Part model, mm, in its own coordinate system. Face numbers are marked on the shaded views. A direction names the side the tool comes from. Coordinates: 2 decimals unless noted, no trailing zeros. Order: outer loops, then holes, each group sorted by start corner. A loop starts at its lowest first (then second) coordinate and runs counter-clockwise, first axis right, second up.
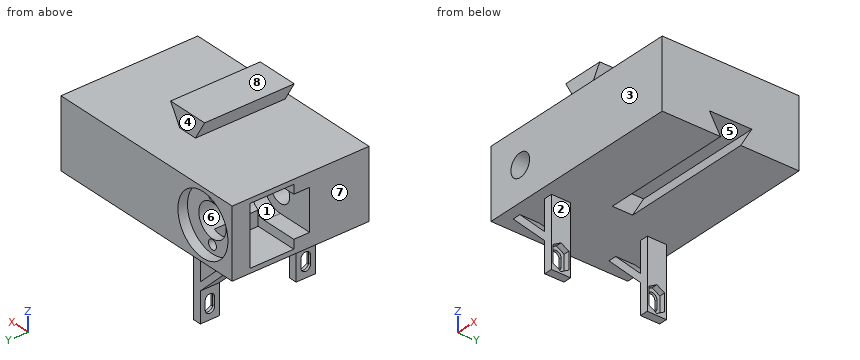
```python
from build123d import *

# Parameters (mm, degrees)
SKETCH1_W                       = 38
SKETCH1_H                       = 50
BOSS_EXTRUDE1_DEPTH             = 25
BOSS_EXTRUDE2_START             = -22.75
BOSS_EXTRUDE2_DEPTH             = 32.75
CUT_EXTRUDE1_DEPTH              = 10
CUT_EXTRUDE2_REACH              = 88.168
CUT_EXTRUDE2_DIRECTION_2_DEPTH  = 87.168439698
SKETCH15_R                      = 11.1
CUT_EXTRUDE8_DEPTH              = 3.5
SKETCH16_R                      = 6.05
CUT_EXTRUDE9_DEPTH              = 19
SKETCH17_R                      = 6.05
CUT_EXTRUDE10_DEPTH             = 5.8
CUT_EXTRUDE11_START             = -16
CUT_EXTRUDE11_DEPTH             = 16
SKETCH19_R                      = 1.75
CUT_EXTRUDE12_DEPTH             = 19
CIRPATTERN1_COUNT               = 2
CIRPATTERN1_ANGLE               = 90
CIRPATTERN1_THE_OTHER_WAY_COUNT = 2
CIRPATTERN1_THE_OTHER_WAY_ANGLE = 90
SKETCH20_R                      = 4.15
CUT_EXTRUDE13_DEPTH             = 58.174207472
SKETCH21_R                      = 1.75
CUT_EXTRUDE14_DEPTH             = 16
SKETCH22_W                      = 3
SKETCH22_H                      = 7
BOSS_EXTRUDE5_DEPTH             = 25
CUT_EXTRUDE15_DEPTH             = 10
CUT_EXTRUDE16_START             = 2.1
CUT_EXTRUDE16_DEPTH             = 2.1
BOSS_EXTRUDE7_DEPTH             = 7
BOSS_EXTRUDE8_DEPTH             = 7


with BuildPart() as part:
    # Sketch1 → Boss-Extrude1 (new body)
    with BuildSketch(Plane.XY):
        with Locations((-19, 0)):
            Rectangle(SKETCH1_W, SKETCH1_H)
    boss_extrude1 = extrude(amount=BOSS_EXTRUDE1_DEPTH)

    # Sketch2 → Boss-Extrude2 (add)
    with BuildSketch(Plane(origin=(0, 0, 0), x_dir=(0, 0, -1), z_dir=(0, 1, 0)).offset(BOSS_EXTRUDE2_START)):
        Polygon((-25, 0), (-25, 3.5), (-32, 7.541451884), (-32, 0), align=None)
    boss_extrude2 = extrude(amount=BOSS_EXTRUDE2_DEPTH)

    # Sketch3 → Cut-Extrude1 (cut)
    with BuildSketch(Plane(origin=(0, 0, 0), x_dir=(0, 0, -1), z_dir=(1, 0, 0))):
        Polygon((0, -3.7), (0, 3.7), (-7, 7.741451884), (-7, -7.741451884), align=None)
    cut_extrude1 = extrude(amount=-CUT_EXTRUDE1_DEPTH, mode=Mode.SUBTRACT)

    # Mirror1: Boss-Extrude1, Boss-Extrude2, Cut-Extrude1 across plane
    add(boss_extrude1.mirror(Plane(origin=(0, 0, 0), x_dir=(0, 0, 1), z_dir=(1, 0, 0))))
    add(boss_extrude2.mirror(Plane(origin=(0, 0, 0), x_dir=(0, 0, 1), z_dir=(1, 0, 0))))
    add(cut_extrude1.mirror(Plane(origin=(0, 0, 0), x_dir=(0, 0, 1), z_dir=(1, 0, 0))), mode=Mode.SUBTRACT)

    # Sketch4 → Cut-Extrude2 (cut, up to next)
    with BuildSketch(Plane(origin=(38, 0, 0), x_dir=(0, 0, -1), z_dir=(1, 0, 0)), mode=Mode.PRIVATE) as cut_extrude2_sk1:
        Polygon((0, -3.7), (0, 3.7), (-7, 7.741451884), (-7, -7.741451884), align=None)
    cut_extrude2_tool1 = extrude(cut_extrude2_sk1.sketch, amount=-CUT_EXTRUDE2_REACH, mode=Mode.PRIVATE) & part.part
    add(cut_extrude2_tool1.solids().sort_by_distance((38, 0, 3.9121))[0], mode=Mode.SUBTRACT)

    # Sketch4 → Cut-Extrude2 direction 2 (cut)
    with BuildSketch(Plane(origin=(38, 0, 0), x_dir=(0, 0, -1), z_dir=(1, 0, 0))):
        Polygon((0, -3.7), (0, 3.7), (-7, 7.741451884), (-7, -7.741451884), align=None)
    extrude(amount=CUT_EXTRUDE2_DIRECTION_2_DEPTH, mode=Mode.SUBTRACT)

    # Sketch15 → Cut-Extrude8 (cut)
    with BuildSketch(Plane(origin=(0, 25, 0), x_dir=(1, 0, 0), z_dir=(0, 1, 0))):
        with Locations(Location((-25, -12.5, 0), (0, 0, 270))):
            Circle(SKETCH15_R)
    extrude(amount=-CUT_EXTRUDE8_DEPTH, mode=Mode.SUBTRACT)

    # Sketch16 → Cut-Extrude9 (cut)
    with BuildSketch(Plane(origin=(0, 21.5, 0), x_dir=(1, 0, 0), z_dir=(0, 1, 0))):
        with Locations(Location((-25, -12.5, 0), (0, 0, 270))):
            Circle(SKETCH16_R)
    extrude(amount=-CUT_EXTRUDE9_DEPTH, mode=Mode.SUBTRACT)

    # Sketch17 → Cut-Extrude10 (cut)
    # profile 1 of 2: a face of its own
    with BuildSketch(Plane(origin=(0, 2.5, 0), x_dir=(1, 0, 0), z_dir=(0, 1, 0))):
        with BuildLine():
            ThreePointArc((-25, -20), (-17.5, -12.5), (-25, -5))
            Line((-25, -5), (-38, -5))
            Line((-38, -5), (-38, -20))
            Line((-38, -20), (-25, -20))
        make_face()
        with Locations(Location((-25, -12.5, 0), (0, 0, 270))):
            Circle(SKETCH17_R, mode=Mode.SUBTRACT)
    # profile 2 of 2: a face of its own
    with BuildSketch(Plane(origin=(0, 2.5, 0), x_dir=(1, 0, 0), z_dir=(0, 1, 0))):
        with Locations(Location((-25, -12.5, 0), (0, 0, 270))):
            Circle(SKETCH17_R)
    extrude(amount=-CUT_EXTRUDE10_DEPTH, mode=Mode.SUBTRACT)

    # Sketch18 → Cut-Extrude11 (cut)
    with BuildSketch(Plane.XZ.offset(-2.5).offset(CUT_EXTRUDE11_START)):
        with BuildLine():
            Line((-25, 18.55), (-38, 18.55))
            Line((-38, 18.55), (-38, 6.45))
            Line((-38, 6.45), (-25, 6.45))
            ThreePointArc((-25, 6.45), (-18.95, 12.5), (-25, 18.55))
        make_face()
    extrude(amount=CUT_EXTRUDE11_DEPTH, mode=Mode.SUBTRACT)

    # Sketch19 → Cut-Extrude12 (cut)
    with BuildSketch(Plane(origin=(0, 21.5, 0), x_dir=(1, 0, 0), z_dir=(0, 1, 0))):
        with Locations(Location((-33, -12.5, 0), (0, 0, 270))):
            Circle(SKETCH19_R)
    cut_extrude12 = extrude(amount=-CUT_EXTRUDE12_DEPTH, mode=Mode.SUBTRACT)

    # CirPattern1: Cut-Extrude12 ×2 about axis
    cirpattern1_axis = Axis((-25, 24.978467243, 12.5), (0, 1, 0))
    for i in range(1, CIRPATTERN1_COUNT):
        add(cut_extrude12.rotate(cirpattern1_axis, i * CIRPATTERN1_ANGLE / (CIRPATTERN1_COUNT - 1)), mode=Mode.SUBTRACT)

    # CirPattern1 the other way: Cut-Extrude12 ×2 about axis
    cirpattern1_the_other_way_axis = Axis((-25, 24.978467243, 12.5), (0, -1, 0))
    for i in range(1, CIRPATTERN1_THE_OTHER_WAY_COUNT):
        add(cut_extrude12.rotate(cirpattern1_the_other_way_axis, i * CIRPATTERN1_THE_OTHER_WAY_ANGLE / (CIRPATTERN1_THE_OTHER_WAY_COUNT - 1)), mode=Mode.SUBTRACT)

    # Sketch20 → Cut-Extrude13 (cut, through all)
    with BuildSketch(Plane(origin=(0, -3.3, 0), x_dir=(1, 0, 0), z_dir=(0, 1, 0))):
        with Locations(Location((-25, -12.5, 0), (0, 0, 270))):
            Circle(SKETCH20_R)
    extrude(amount=-CUT_EXTRUDE13_DEPTH, mode=Mode.SUBTRACT)

    # Sketch21 → Cut-Extrude14 (cut)
    with BuildSketch(Plane.XZ.offset(-18.5)):
        with BuildLine():
            Line((-38, 6.45), (-38, 1.7))
            Line((-38, 1.7), (-22.2, 1.7))
            Line((-22.2, 1.7), (-22.2, 23.3))
            Line((-22.2, 23.3), (-38, 23.3))
            Line((-38, 23.3), (-38, 18.55))
            Line((-38, 18.55), (-25, 18.55))
            ThreePointArc((-25, 18.55), (-31.05, 12.5), (-25, 6.45))
            Line((-25, 6.45), (-38, 6.45))
        make_face()
        with Locations(Location((-25, 4.5, 0), (0, 0, 180))):
            Circle(SKETCH21_R, mode=Mode.SUBTRACT)
        with Locations((-25, 20.5)):
            Circle(SKETCH21_R, mode=Mode.SUBTRACT)
    extrude(amount=CUT_EXTRUDE14_DEPTH, mode=Mode.SUBTRACT)

    # Sketch22 → Boss-Extrude5 (add)
    with BuildSketch(Plane(origin=(0, 0, 0), x_dir=(-1, 0, 0), z_dir=(0, 0, -1))):
        with Locations((17.5, 17.5)):
            Rectangle(SKETCH22_W, SKETCH22_H)
        with Locations((17.5, -17.5)):
            Rectangle(SKETCH22_W, SKETCH22_H)
    extrude(amount=BOSS_EXTRUDE5_DEPTH)

    # Sketch23 → Cut-Extrude15 (cut)
    with BuildSketch(Plane.ZY.offset(19)):
        with BuildLine():
            Line((-18.05, 19.25), (-21.05, 19.25))
            ThreePointArc((-21.05, 19.25), (-22.8, 17.5), (-21.05, 15.75))
            Line((-21.05, 15.75), (-18.05, 15.75))
            ThreePointArc((-18.05, 15.75), (-16.3, 17.5), (-18.05, 19.25))
        make_face()
        with BuildLine():
            Line((-18.05, -15.75), (-21.05, -15.75))
            ThreePointArc((-21.05, -15.75), (-22.8, -17.5), (-21.05, -19.25))
            Line((-21.05, -19.25), (-18.05, -19.25))
            ThreePointArc((-18.05, -19.25), (-16.3, -17.5), (-18.05, -15.75))
        make_face()
    extrude(amount=-CUT_EXTRUDE15_DEPTH, mode=Mode.SUBTRACT)

    # Sketch24 → Cut-Extrude16 (cut)
    with BuildSketch(Plane.ZY.offset(16).offset(CUT_EXTRUDE16_START)):
        with BuildLine():
            Line((-21.05, 19.25), (-20.330533563, 19.25))
            Line((-20.330533563, 19.25), (-19.695448267, 20.35))
            Line((-19.695448267, 20.35), (-22.695448267, 20.35))
            Line((-22.695448267, 20.35), (-24.340896534, 17.5))
            Line((-24.340896534, 17.5), (-22.695448267, 14.65))
            Line((-22.695448267, 14.65), (-19.695448267, 14.65))
            Line((-19.695448267, 14.65), (-20.330533563, 15.75))
            Line((-20.330533563, 15.75), (-21.05, 15.75))
            ThreePointArc((-21.05, 15.75), (-22.8, 17.5), (-21.05, 19.25))
        make_face()
        with BuildLine():
            Line((-19.404551733, 20.35), (-18.769466437, 19.25))
            Line((-18.769466437, 19.25), (-18.05, 19.25))
            ThreePointArc((-18.05, 19.25), (-16.3, 17.5), (-18.05, 15.75))
            Line((-18.05, 15.75), (-18.769466437, 15.75))
            Line((-18.769466437, 15.75), (-19.404551733, 14.65))
            Line((-19.404551733, 14.65), (-16.404551733, 14.65))
            Line((-16.404551733, 14.65), (-14.759103466, 17.5))
            Line((-14.759103466, 17.5), (-16.404551733, 20.35))
            Line((-16.404551733, 20.35), (-19.404551733, 20.35))
        make_face()
        Polygon((-20.330533563, 19.25), (-18.769466437, 19.25), (-19.404551733, 20.35), (-19.695448267, 20.35), align=None)
        Polygon((-19.404551733, 14.65), (-18.769466437, 15.75), (-20.330533563, 15.75), (-19.695448267, 14.65), align=None)
        Polygon((-19.404551733, -20.35), (-17.759103466, -17.5), (-19.404551733, -14.65), (-19.695448267, -14.65), (-21.340896534, -17.5), (-19.695448267, -20.35), align=None)
        Polygon((-21.340896534, -17.5), (-19.695448267, -14.65), (-22.695448267, -14.65), (-24.340896534, -17.5), (-22.695448267, -20.35), (-19.695448267, -20.35), align=None)
        with BuildLine():
            Line((-19.404551733, -14.65), (-18.769466437, -15.75))
            Line((-18.769466437, -15.75), (-18.05, -15.75))
            ThreePointArc((-18.05, -15.75), (-16.3, -17.5), (-18.05, -19.25))
            Line((-18.05, -19.25), (-18.769466437, -19.25))
            Line((-18.769466437, -19.25), (-19.404551733, -20.35))
            Line((-19.404551733, -20.35), (-16.404551733, -20.35))
            Line((-16.404551733, -20.35), (-14.759103466, -17.5))
            Line((-14.759103466, -17.5), (-16.404551733, -14.65))
            Line((-16.404551733, -14.65), (-19.404551733, -14.65))
        make_face()
    extrude(amount=-CUT_EXTRUDE16_DEPTH, mode=Mode.SUBTRACT)

    # Sketch26 → Boss-Extrude7 (add)
    with BuildSketch(Plane.XZ.offset(21)):
        Polygon((-19, -14), (-33, 0), (-30, 0), (-19, -11), align=None)
    extrude(amount=-BOSS_EXTRUDE7_DEPTH)

    # Sketch28 → Boss-Extrude8 (add)
    with BuildSketch(Plane(origin=(0, 21, 0), x_dir=(1, 0, 0), z_dir=(0, 1, 0))):
        Polygon((-33, 0), (-30, 0), (-19, 11), (-19, 14), align=None)
    extrude(amount=-BOSS_EXTRUDE8_DEPTH)


solid = part.part
```
(1) Slice it at D-D, the plane y = 5. Give the cut face in (x, z).
(2) Slice it at B-B, the plane y = -1.5. Give the cut face in (x, z).
(3) Slice it at C-C, the plane z = 26. Give the cut face in (x, y), then the cut area to 3 significant figures.
(4) Slice it at A-A, the plane x = 33. Give the cut face in (y, z), then the cut area to 3 significant figures.
(5) Drop flat-ended pins along their axis: pin 1 (3 mm diameter, centred on y = 13.5, z = -16.5, fed in from +X); pin 2 (18.5 mm diameter, centred on x = -24, z = -17.5, fed in from -Y); pin 3 (6 mm diameter, centred on y = 8, z = 19.5, fed in from -X); pin 4 (12 mm diameter, centred on x = 12, z = -10.5, fed in from +Y). Give the stop position or say it passes through.
(6) Pull direction X, two halves, no side cores. Call the marked faces 6, 7 and 8: +X half, -X half, draft (parallel to the pull), parting line (faces both ways), or undercut.
(7) Tool access for the marked faces 1, 2, 3, 4 and 5: list every direction of +Z, -Z, +X, -X, +Y, -Y with a clear straight run to the whole face (end or side of a thin tool).
(8) Probe line 1 (X direction, y = 23, z = 12); line 2 (Z direction, x = -34, y = -2); line 3 (Z direction, x = 4, y = 7.5). List the from-to ranges inside material, lowest first.
Here are the results:
1. outline: (-38, 0) - (38, 0) - (38, 2.25) - (-10, 2.25) - (-10, 7) - (38, 7) - (38, 25) - (3.5, 25) - (7.54, 32) - (-7.54, 32) - (-3.5, 25) - (-38, 25) - (-38, 23.3) - (-22.2, 23.3) - (-22.2, 17.86) arc R6.05 cw to (-22.2, 7.14) - (-22.2, 1.7) - (-38, 1.7) - close
2. outline: (-38, 0) - (-10, 0) - (-10, 7) - (38, 7) - (38, 25) - (3.5, 25) - (7.54, 32) - (-7.54, 32) - (-3.5, 25) - (-38, 25) - (-38, 20) - (-25, 20) arc R7.5 cw to (-25, 5) - (-38, 5) - close
3. outline: (-4.08, -22.75) - (4.08, -22.75) - (4.08, 10) - (-4.08, 10) - close
3. area: 267 mm2
4. outline: (-25, 0) - (-3.7, 0) - (-7.74, 7) - (7.74, 7) - (3.7, 0) - (25, 0) - (25, 25) - (-25, 25) - close
4. area: 1,170 mm2
5. pin 1: stops at x = -16
5. pin 2: stops at y = -21
5. pin 3: stops at x = -22.2
5. pin 4: passes through
6. face 6: undercut
6. face 7: -X half
6. face 8: draft
7. face 1: -X
7. face 2: -Z, +X, +Y, -Y
7. face 3: +Z, -Z, +X, -X, -Y
7. face 4: +Z, +X, -X, +Y
7. face 5: +X
8. line 1: x = -38 to -36.09, -13.91 to 38
8. line 2: z = 0 to 5, 20 to 25
8. line 3: z = 0 to 6.58, 7 to 25, 25.87 to 32
